For this review, take the finished solid that the model builds, in its own axes (mm). Coordinates: 2 decimals unless noted, no trailing zeros. Loops run counter-clockwise (first coordinate to the right, second up) from the corner with the lowest first, then second, coordinate; pieces in that order, holes last. Notation, with made-up numbers: (-5.5, 38) -> (12.5, 38) arc R31 cw to (12.5, 68) -> close; hole circle Ø6 at (62, 45). An arc over 180 degrees is marked (long way). One line per item, written item: value.
from build123d import *

# Parameters (mm, degrees)
SKETCH1_W           = 140
SKETCH1_H           = 150
BOSS_EXTRUDE1_DEPTH = 5
SKETCH2_R           = 4.05
CUT_EXTRUDE1_DEPTH  = 103.713192921
FILLET1_R           = 4


with BuildPart() as part:
    # Sketch1 → Boss-Extrude1 (new body)
    with BuildSketch(Plane(origin=(0, 0, 0), x_dir=(1, 0, 0), z_dir=(0, 1, 0))):
        Rectangle(SKETCH1_W, SKETCH1_H)
    extrude(amount=BOSS_EXTRUDE1_DEPTH)

    # Sketch2 → Cut-Extrude1 (cut, through all)
    with BuildSketch(Plane(origin=(0, 5, 0), x_dir=(1, 0, 0), z_dir=(0, 1, 0))):
        with Locations(Location((-25, 0, 0), (0, 0, 270))):
            Circle(SKETCH2_R)
    cut_extrude1 = extrude(amount=-CUT_EXTRUDE1_DEPTH, mode=Mode.SUBTRACT)

    # Mirror1: Cut-Extrude1 across plane
    add(cut_extrude1.mirror(Plane(origin=(0, 0, 0), x_dir=(0, 0, 1), z_dir=(1, 0, 0))), mode=Mode.SUBTRACT)

    # Fillet1
    fillet1_edges = [part.edges().sort_by_distance(p)[0] for p in [
        (70, 2.5, 75),
        (-70, 2.5, 75),
        (-70, 2.5, -75),
        (70, 2.5, -75),
    ]]
    fillet(fillet1_edges, radius=FILLET1_R)


solid = part.part
1. To check wall thickness, follow probe 1 along X at (y, z) = (1.15, 0); probe 2 along Z at (x, y) = (-23.5, 2.2). State the ranges of each line that lie inside material, in increasing order. Write a range as from..to.
Return value:
probe 1: x = -70..-29.05, -20.95..20.95, 29.05..70
probe 2: z = -75..-3.76, 3.76..75
2. The part is to be moulded in two halves that separate along Z. For faces 1 (the flat face through (-1, 2, 75)), 2 (the cylindrical face through (28.954, 2.535, -0.878)), 3 (the flat face through (-70, 2, 1)), say which applies: pulls with the +Z half, pulls with the -Z half, needs draft (parallel to the pull), parting line crosses it, or undercut.
Return value:
face 1: pulls with the +Z half
face 2: undercut
face 3: needs draft
3. Take a section at B-B, the plane z = 0. Give the boundary of the cut face in (x, y), and give its area (3 significant figures).
Return value:
outline: (-70, 0) -> (-29.05, 0) -> (-29.05, 5) -> (-70, 5) -> close; (-20.95, 0) -> (20.95, 0) -> (20.95, 5) -> (-20.95, 5) -> close; (29.05, 0) -> (70, 0) -> (70, 5) -> (29.05, 5) -> close
area: 619 mm2
4. Take a section at A-A, the plane x = 25. Give the boundary of the cut face in (y, z), and give its area (4 significant figures).
Return value:
outline: (0, -75) -> (5, -75) -> (5, -4.05) -> (0, -4.05) -> close; (0, 4.05) -> (5, 4.05) -> (5, 75) -> (0, 75) -> close
area: 709.5 mm2
